Read the model definition and answer for the solid it produces. Units are mm, in the model's axes. A direction names the side the tool comes from. Give positions to 0.01 mm unless a question says otherwise; leave off trailing zeros. Order: outer loops, then holes, each group sorted by start corner. A loop starts at its lowest first (then second) coordinate and runs counter-clockwise, first axis right, second up. Notation, with made-up numbers: (68, 0.5) - (85, 0.5) arc R32 cw to (85, 39.5) - close; hole circle Ø9 at (42.5, 22.25). An arc over 180 degrees is marked (long way). Return JSON: item names as keys, results as strings.
```python
from build123d import *

# Parameters (mm, degrees)
SKETCH1_W           = 57
SKETCH1_H           = 57
BOSS_EXTRUDE1_DEPTH = 76
SKETCH3_R           = 2.5
CUT_EXTRUDE1_DEPTH  = 77
CUT_EXTRUDE2_DEPTH  = 77
SKETCH5_OUTSIDE_W   = 81.158
SKETCH5_OUTSIDE_H   = 81.158
CUT_EXTRUDE3_DEPTH  = 71.2
SKETCH6_R           = 19.05
BOSS_EXTRUDE2_DEPTH = 1.6


with BuildPart() as part:
    # Sketch1 → Boss-Extrude1 (new body)
    with BuildSketch(Plane.XY):
        Rectangle(SKETCH1_W, SKETCH1_H)
    extrude(amount=-BOSS_EXTRUDE1_DEPTH)

    # Sketch3 → Cut-Extrude1 (cut, through all)
    with BuildSketch(Plane(origin=(0, 0, -76), x_dir=(-1, 0, 0), z_dir=(0, 0, -1))):
        with Locations((-23.57, 23.57)):
            Circle(SKETCH3_R)
        with Locations((-23.57, -23.57)):
            Circle(SKETCH3_R)
        with Locations((23.57, 23.57)):
            Circle(SKETCH3_R)
        with Locations((23.57, -23.57)):
            Circle(SKETCH3_R)
    extrude(amount=-CUT_EXTRUDE1_DEPTH, mode=Mode.SUBTRACT)

    # Sketch4 → Cut-Extrude2 (cut, through all)
    with BuildSketch(Plane(origin=(0, 0, -76), x_dir=(-1, 0, 0), z_dir=(0, 0, -1))):
        with BuildLine():
            Line((-28.5, 23.57), (-28.5, 28.5))
            Line((-28.5, 28.5), (-23.57, 28.5))
            ThreePointArc((-23.57, 28.5), (-27.056036431, 27.056036431), (-28.5, 23.57))
        make_face()
        with BuildLine():
            Line((23.57, 28.5), (28.5, 28.5))
            Line((28.5, 28.5), (28.5, 23.57))
            ThreePointArc((28.5, 23.57), (27.056036431, 27.056036431), (23.57, 28.5))
        make_face()
        with BuildLine():
            Line((-28.5, -23.57), (-28.5, -28.5))
            Line((-28.5, -28.5), (-23.57, -28.5))
            ThreePointArc((-23.57, -28.5), (-27.056036431, -27.056036431), (-28.5, -23.57))
        make_face()
        with BuildLine():
            Line((23.57, -28.5), (28.5, -28.5))
            Line((28.5, -28.5), (28.5, -23.57))
            ThreePointArc((28.5, -23.57), (27.056036431, -27.056036431), (23.57, -28.5))
        make_face()
    extrude(amount=-CUT_EXTRUDE2_DEPTH, mode=Mode.SUBTRACT)

    # Sketch5 outside → Cut-Extrude3 (cut)
    with BuildSketch(Plane(origin=(0, 0, -76), x_dir=(-1, 0, 0), z_dir=(0, 0, -1))):
        Rectangle(SKETCH5_OUTSIDE_W, SKETCH5_OUTSIDE_H)
        with BuildLine():
            Line((-28.5, 13.71), (-28.5, -13.71))
            ThreePointArc((-28.5, -13.71), (-27.056036431, -17.196036431), (-23.57, -18.64))
            ThreePointArc((-23.57, -18.64), (-20.083963569, -20.083963569), (-18.64, -23.57))
            ThreePointArc((-18.64, -23.57), (-17.196036431, -27.056036431), (-13.71, -28.5))
            Line((-13.71, -28.5), (13.71, -28.5))
            ThreePointArc((13.71, -28.5), (17.196036431, -27.056036431), (18.64, -23.57))
            ThreePointArc((18.64, -23.57), (20.083963569, -20.083963569), (23.57, -18.64))
            ThreePointArc((23.57, -18.64), (27.056036431, -17.196036431), (28.5, -13.71))
            Line((28.5, -13.71), (28.5, 13.71))
            ThreePointArc((28.5, 13.71), (27.056036431, 17.196036431), (23.57, 18.64))
            ThreePointArc((23.57, 18.64), (20.083963569, 20.083963569), (18.64, 23.57))
            ThreePointArc((18.64, 23.57), (17.196036431, 27.056036431), (13.71, 28.5))
            Line((13.71, 28.5), (-13.71, 28.5))
            ThreePointArc((-13.71, 28.5), (-17.196036431, 27.056036431), (-18.64, 23.57))
            ThreePointArc((-18.64, 23.57), (-20.083963569, 20.083963569), (-23.57, 18.64))
            ThreePointArc((-23.57, 18.64), (-27.056036431, 17.196036431), (-28.5, 13.71))
        make_face(mode=Mode.SUBTRACT)
    extrude(amount=-CUT_EXTRUDE3_DEPTH, mode=Mode.SUBTRACT)

    # Sketch6 → Boss-Extrude2 (add)
    with BuildSketch(Plane.XY):
        Circle(SKETCH6_R)
    extrude(amount=BOSS_EXTRUDE2_DEPTH)


solid = part.part
```
Q1. A cutting plane is placed at A-A (z = -57). Write down the section's boundary in (x, y), and give its area (3 significant figures).
Values:
{"outline": "(-28.5, -13.71) arc R4.93 ccw to (-23.57, -18.64) arc R4.93 cw to (-18.64, -23.57) arc R4.93 ccw to (-13.71, -28.5) - (13.71, -28.5) arc R4.93 ccw to (18.64, -23.57) arc R4.93 cw to (23.57, -18.64) arc R4.93 ccw to (28.5, -13.71) - (28.5, 13.71) arc R4.93 ccw to (23.57, 18.64) arc R4.93 cw to (18.64, 23.57) arc R4.93 ccw to (13.71, 28.5) - (-13.71, 28.5) arc R4.93 ccw to (-18.64, 23.57) arc R4.93 cw to (-23.57, 18.64) arc R4.93 ccw to (-28.5, 13.71) - close", "area": "2,840 mm²"}
Q2. Given pin 1 (7.5 mm diameter, centred on x = 21.5, y = -22.5, fed in from -Z); pin 2 (10 mm diameter, centred on x = -17, y = 18, fed in from +Z); pin 3 (1.5 mm diameter, centred on y = 15.5, z = -23, fed in from -X); pin 4 (7.5 mm diameter, centred on x = -24, y = -22.5, fed in from -Z), each flat-ended and moving along its own axis, determine where each tip first touches the part or whether it passes through.
Values:
{"pin 1": "stops at z = -76", "pin 2": "stops at z = 0", "pin 3": "stops at x = -28.39", "pin 4": "stops at z = -4.8"}
Q3. Consider L1, parallel to Y at x = 23.57, z = -1.7; L2, parallel to X at y = -23, z = -3; L3, parallel to Z at x = -21, y = 25. Determine where each line is inside the solid, lowest interval first.
Values:
{"L1": "y = -28.5 to -26.07, -21.07 to 21.07, 26.07 to 28.5", "L2": "x = -28.5 to -26, -21.14 to 21.14, 26 to 28.5", "L3": "z = -4.8 to 0"}
Q4. For faces 1 (the cylindrical face through (-15.12, -11.59, 0.79)), 2 (the flat face through (24.5, -21, -4.8)), 3 (the flat face through (-21, 24.5, -4.8)), determine the directions among +Z, -Z, +X, -X, +Y, -Y from which every point of the face is accessible in a straight line to the end or side of a thin tool.
Values:
{"face 1": "+Z", "face 2": "-Z, +X, -Y", "face 3": "-Z, -X, +Y"}
Q5. Determine the mould class of faces 4 (the cylindrical face through (-27.09, 27.02, -2.43)), 5 (the cylindrical face through (-21.586, -25.091, -2.434)), 6 (the cylindrical face through (27.02, 27.09, -2.43)), 7 (the flat face through (-21.6, -25.5, -4.8)) for opening direction X: released by +X, released by -X, zero draft, split by the parting line, or undercut.
Values:
{"face 4": "released by -X", "face 5": "undercut", "face 6": "released by +X", "face 7": "zero draft"}
